Geometry: final body of the model. Coordinates: model frame, mm. A direction names the side the tool comes from. Give positions to 0.01 mm unless a question says otherwise; leave off trailing zeros. Write each loop counter-clockwise with the first axis right and the second up, starting at its lowest first coordinate (ties: lowest second). Pieces come first, ordered by that corner, then holes. Notation, with made-up numbers: M 79.5,-7.5 L 84.5,-7.5 A12 ccw 84.5,1.5 Z; hole C -10.75,5 d3. An arc over 180 degrees is marked long. Use a Markdown table: item, result. Add a question column.
1) Section A-A on y = 0. Return the cut outline in (x, z) (3 decimals).
2) Section B-B on y = 10. Return the cut outline in (x, z).
3) Set-up query: faces 5 (the flat face through (20, 11.43, -2)), 6 (the flat face through (3.828, 3.792, 2.23)), 7 (the cylindrical face through (-1.447, 10.822, -0.089)). Return all of +Z, -Z, +X, -X, +Y, -Y with unobstructed straight access to the full face (end or side cutting, diameter ignored); none if empty.
4) Pin query (flat end, axial travel): pin 1 (1 mm diameter, centred on y = 2.5, z = 4.5, fed in from +X); pin 2 (6 mm diameter, centred on x = 18.034, z = 0, fed in from -Y); pin 3 (3 mm diameter, centred on x = 6.5, z = 4.5, fed in from +Y). Return the tip coordinate at first contact, or that it passes through.
5) Line query: line 1 (Z direction, x = 4.75, y = -2.5); line 2 (X direction, y = 2.5, z = -4.25); line 3 (Y direction, x = 1.4, z = 0) (3 decimals). Output: solid intervals per line, ascending.
6) Draft query along Z for faces 1 (the flat face through (3.828, 3.828, -2.169)), 2 (the flat face through (6, 7, -6.35)), 3 (the flat face through (15, 6.35, 0)), 4 (the flat face through (2.54, -2.2, 0.1)). Return one class per face: +Z half, -Z half, draft (parallel to the pull), parting line (faces both ways), or undercut.
7) Section C-C on z = 0.75. State how many separate pieces and enclosed holes the cut face has, then the cut area to 3 significant figures.
8) Section D-D on y = -6.5. Return the cut outline in (x, z), then the cut area to 3 significant figures.
Autodesk Inventor part; units mm, degrees
ref_plane "YZ Plane" through (0, 0, 0) normal (1, 0, 0) x (0, 1, 0)
ref_plane "XZ Plane" through (0, 0, 0) normal (0, 1, 0) x (-1, 0, 0)
ref_plane "XY Plane" through (0, 0, 0) normal (0, 0, 1) x (1, 0, 0)
sketch "Sketch1" plane through (0, 0, 0) normal (1, 0, 0) x (0, 1, 0)
  circle A0 centre (0, 0) radius 1.905
  line L0 (0, 0) -> (0, -6.35)
  line L1 (0, 0) -> (0, 6.35)
  line L2 (0, 6.35) -> (-6.35, 6.35)
  line L3 (0, -6.35) -> (6.35, -6.35)
  line L4 (-6.35, 6.35) -> (6.35, 6.35)
  line L5 (6.35, 6.35) -> (6.35, -6.35)
  line L6 (6.35, -6.35) -> (-6.35, -6.35)
  line L7 (-6.35, -6.35) -> (-6.35, 6.35)
  dimension "d0" = 3.81
  dimension "d2" = 6.35
  dimension "d3" = 6.35
  dimension "d4" = 6.35
  dimension "d5" = 6.35
extrude "Extrusion1" add sketch "Sketch1" along normal blind 5.08 contours A0 L1 L4 L5 L3 L0 | A0 L0 L6 L7 L2 L1
sketch "Sketch2" plane through (5.08, 0, 0) normal (1, 0, 0) x (0, 0, -1)
  point P0 (0, 0)
sketch "Sketch3" plane through (5.08, 0, 0) normal (1, 0, 0) x (0, 0, -1)
  line L0 (0, 0) -> (0, -5.08)
  arc A0 (0, -5.08) -> (0, 0) centre (-4.3994, -2.54) ccw
  line L1 (4.3994, -2.54) -> (0, -5.08)
  line L2 (0, -5.08) -> (-4.3994, -2.54)
  line L3 (-4.3994, 2.54) -> (0, 5.08)
  line L4 (4.3994, 2.54) -> (4.3994, -2.54)
  line L5 (-4.3994, -2.54) -> (-4.3994, 2.54)
  line L6 (0, 5.08) -> (4.3994, 2.54)
  dimension "d8" = 5.08
extrude "Extrusion2" cut sketch "Sketch3" against normal blind 2.54 contours A0 L0 | L2 L5 L3 L6 L4 L1
sketch "Sketch4" plane through (0, -6.35, -6.35) normal (0, -1, 0) x (1, 0, 0)
  line L0 (0, 12.7) -> (5.08, 12.7)
  line L1 (0, 0) -> (5.08, 0)
  line L2 (5.08, 12.7) -> (0, 12.7)
  line L3 (0, 12.7) -> (0, 0)
  line L4 (0, 0) -> (5.08, 0)
  line L5 (5.08, 0) -> (5.08, 12.7)
  point P0 (0, 6.35)
extrude "Extrusion3" add sketch "Sketch4" along normal blind 2.54
sketch "Sketch5" plane through (0, 6.35, 6.35) normal (0, 1, 0) x (1, 0, 0)
  line L0 (5.08, 0) -> (0, 0)
  line L1 (5.08, 12.7) -> (5.08, 0)
  line L2 (0, 0) -> (5.08, 0)
  line L3 (5.08, 0) -> (5.08, 12.7)
  line L4 (5.08, 12.7) -> (0, 12.7)
  line L5 (0, 12.7) -> (0, 0)
  point P0 (0, 6.35)
extrude "Extrusion4" add sketch "Sketch5" along normal blind 5.08
sketch "Sketch6" plane through (5.08, 0, 0) normal (1, 0, 0) x (0, 0, -1)
  line L0 (-6.35, -8.89) -> (-6.35, 11.43)
  line L1 (-6.35, 11.43) -> (-6.35, 6.35)
  line L2 (-6.35, -8.89) -> (-6.35, -6.35)
  line L3 (6.35, 11.43) -> (-6.35, 11.43)
  line L4 (-6.35, 6.35) -> (6.35, 6.35)
  line L5 (6.35, 6.35) -> (6.35, 11.43)
  line L6 (6.35, 11.43) -> (-6.35, 11.43)
  line L7 (-6.35, 11.43) -> (-6.35, 6.35)
  line L8 (6.35, -8.89) -> (-6.35, -8.89)
  line L9 (-6.35, -6.35) -> (6.35, -6.35)
  line L10 (6.35, -6.35) -> (6.35, -8.89)
  line L11 (6.35, -8.89) -> (-6.35, -8.89)
  line L12 (-6.35, -8.89) -> (-6.35, -6.35)
  point P0 (0, 0)
  dimension "d15" = 5.08
  dimension "d16" = 2.54
extrude "Extrusion5" add sketch "Sketch6" along normal blind 19.304
sketch "Sketch7" plane through (0, -8.89, -6.35) normal (0, -1, 0) x (1, 0, 0)
  line L0 (24.384, 0) -> (24.384, 12.7)
  line L1 (24.384, 6.35) -> (18.034, 6.35)
  circle A0 centre (18.034, 6.35) radius 2.2606
  point P0 (0, 6.35)
  dimension "d19" = 6.35
  dimension "d20" = 4.5212
extrude "Extrusion6" cut sketch "Sketch7" against normal blind 63.5
sketch "Sketch8" plane through (0, -8.89, 6.35) normal (0, 0, 1) x (1, 0, 0)
  line L0 (0, 0) -> (24.384, 0)
  line L1 (5.08, 2.54) -> (24.384, 2.54)
  line L2 (24.384, 0) -> (5.08, 0)
  line L3 (5.08, 0) -> (5.08, 2.54)
  line L4 (5.08, 2.54) -> (24.384, 2.54)
  line L5 (24.384, 2.54) -> (24.384, 0)
  point P0 (0, 8.89)
extrude "Extrusion7" cut sketch "Sketch8" against normal blind 25.4
sketch "Sketch10" plane through (0, -8.89, 6.35) normal (0, 0, 1) x (1, 0, 0)
  line L0 (5.08, 15.24) -> (0, 15.24)
  line L1 (0, 0) -> (0, 20.32)
  line L2 (0, 15.24) -> (0, 20.32)
  line L3 (0, 20.32) -> (-3.175, 20.32)
  arc A0 (0, 15.24) -> (-3.175, 20.32) centre (-9.8202, 12.6345) ccw
  line L4 (0, 20.32) -> (0, 23.495)
  arc A1 (-3.175, 20.32) -> (0, 23.495) centre (-8.5941, 28.9141) ccw
  line L5 (0, 20.32) -> (12.7, 20.32)
  line L6 (0, 20.32) -> (24.384, 20.32)
  arc A2 (0, 23.495) -> (12.7, 20.32) centre (14.1996, 53.3059) ccw
  point P0 (0, 8.89)
  dimension "d25" = 3.175
  dimension "d26" = 10.16
  dimension "d27" = 3.175
  dimension "d28" = 10.16
  dimension "d29" = 12.7
  dimension "d30" = 33.02
extrude "Extrusion8" add sketch "Sketch10" against normal up to surface (12.7 mm away)
fillet "Fillet1" radius 3.175 2 edges at (0, 14.605, 0) (-3.175, 11.43, 0)
sketch "Sketch11" plane through (0, 0, 0) normal (-1, 0, 0) x (0, 0, 1)
  line L0 (6.35, -8.89) -> (-6.35, -8.89)
  line L1 (-6.35, 8.8491) -> (-6.35, 13.6192)
  line L2 (6.35, -8.89) -> (-6.35, -8.89)
  line L3 (-6.35, -8.89) -> (-6.35, 11.2341)
  line L4 (-6.35, 11.2341) -> (6.35, 11.2341)
  line L5 (6.35, 11.2341) -> (6.35, -8.89)
  point P0 (0, 0)
  point P1 (-6.35, 13.4242)
extrude "Extrusion9" add sketch "Sketch11" along normal blind 1.4732
fillet "Fillet2" radius 3.175 1 edges at (-1.4732, 11.2341, 0)
sketch "Sketch12" plane through (0, 0, 0) normal (1, 0, 0) x (0, 0, -1)
  circle A0 centre (0, 0) radius 1.905
extrude "Extrusion10" cut sketch "Sketch12" against normal blind 18.9357
properties part number "printed piston fitting wings"
Found:
| question | item | result |
|---|---|---|
| 1 | outline | M -1.473,-6.35 L 5.08,-6.35 L 5.08,-4.399 L 2.54,-4.399 L 2.54,-1.905 L -1.473,-1.905 Z; M -1.473,1.905 L 2.54,1.905 L 2.54,4.399 L 5.08,4.399 L 5.08,6.35 L -1.473,6.35 Z |
| 2 | outline | M -1.47,-6.35 L 24.38,-6.35 L 24.38,6.35 L -1.47,6.35 Z; hole C 18.03,0 d4.52 |
| 3 | face 5 | +Z, -Z, +X, +Y |
| 3 | face 6 | +X |
| 3 | face 7 | +Z, -Z, -X, +Y |
| 4 | pin 1 | x = 5.08 |
| 4 | pin 2 | y = 6.35 |
| 4 | pin 3 | y = 12.7 |
| 5 | line 1 | -6.35 to -4.4, 4.4 to 6.35 |
| 5 | line 2 | -1.47 to 2.54 |
| 5 | line 3 | -8.89 to -1.905, 1.905 to 13.604 |
| 6 | face 1 | undercut |
| 6 | face 2 | -Z half |
| 6 | face 3 | draft |
| 6 | face 4 | undercut |
| 7 | separate pieces | 3 |
| 7 | enclosed holes | 0 |
| 7 | area | 186 mm² |
| 8 | outline | M -1.47,-6.35 L 5.08,-6.35 L 5.08,6.35 L -1.47,6.35 Z |
| 8 | area | 83.2 mm² |
